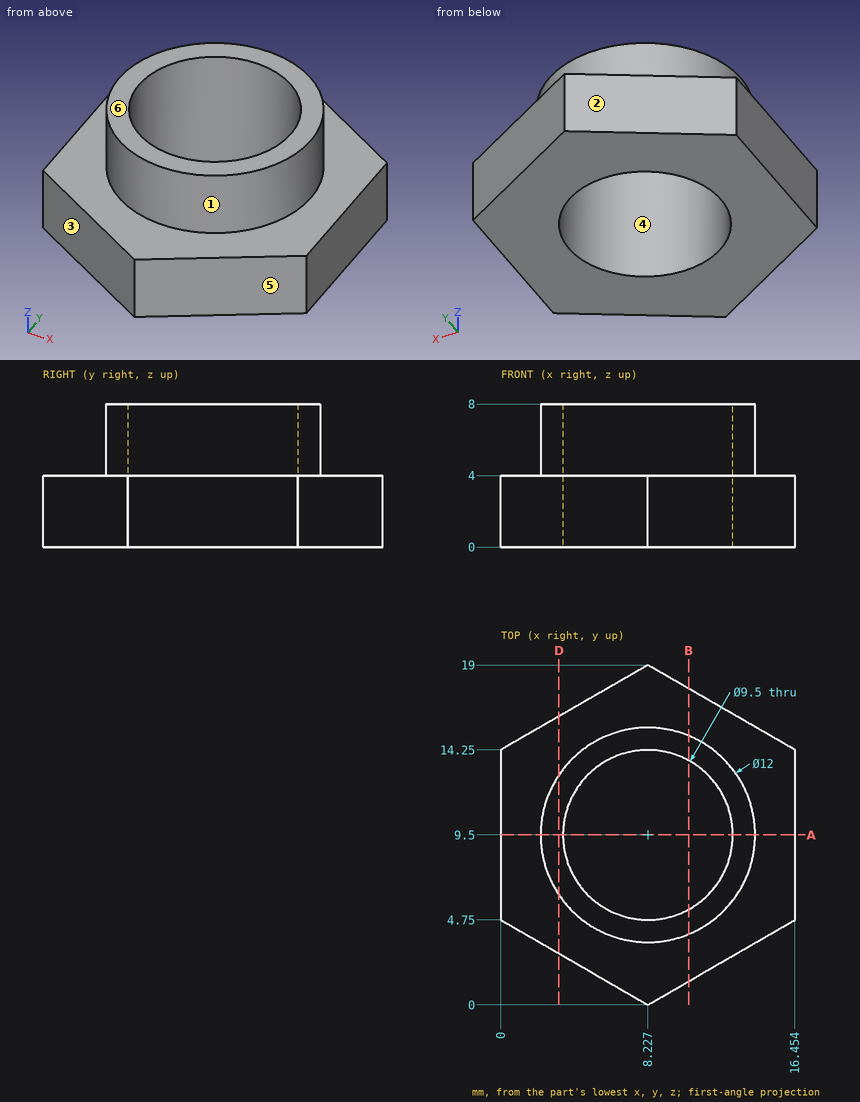
Could you check a few things on this drawing? It's one solid part, dimensions in mm from its lowest x, y, z. A direction names the side the tool comes from. Round coordinates to 2 decimals unless told otherwise and drop trailing zeros. Write each loop counter-clockwise with the first axis right and the second up, starting at its lowest first coordinate (ties: lowest second). Pieces come first, ordered by that corner, then holes.
Q1. Which directions (+Z, -Z, +X, -X, +Y, -Y) give clear straight access to the entire face, cutting with the end or side of a thin tool? Please do the marked faces 1 and 2.
Q2. If we mould it in two halves opening along X, with no side actions, what happens to the marked faces 3, 4, 5 and 6? For each: +X half, -X half, draft (parallel to the pull), parting line (faces both ways), or undercut.
Q3. If we section it at D-D on x = 3.25: Write out the boundary of the cut face in (y, z).
Q4. If we section it at A-A on y = 9.5: Write out the boundary of the cut face in (x, z) (1 decimal).
Q5. If we section it at B-B on x = 10.5: Write out the boundary of the cut face in (y, z).
Q6. Will these pins go through, and if not, where does the flat tip stop? P1, Ø3, axis at x = 9, y = 12, coming from the -Z side; P2, Ø2, axis at x = 13.5, z = 3.5, coming from the +Y side; P3, Ø4, axis at x = 14, y = 12.5, coming from the +Z side; P4, Ø2, axis at x = 12, z = 6.5, coming from the -Y side.
Q7. Please list where these lines run through material, in increasing order: probe 1 along Z at (x, y) = (1.5, 12); probe 2 along Y at (x, z) = (10.5, 2.25); probe 3 along Y at (x, z) = (12.25, 2) (1 decimal).
Answer below:
1. face 1: +Z
1. face 2: +Z, -Z, -X, +Y
2. face 3: -X half
2. face 4: undercut
2. face 5: +X half
2. face 6: draft
3. outline: (2.87, 0) - (16.13, 0) - (16.13, 4) - (12.85, 4) - (12.85, 8) - (6.15, 8) - (6.15, 4) - (2.87, 4) - close
4. outline: (0, 0) - (3.5, 0) - (3.5, 8) - (2.2, 8) - (2.2, 4) - (0, 4) - close; (13, 0) - (16.5, 0) - (16.5, 4) - (14.2, 4) - (14.2, 8) - (13, 8) - close
5. outline: (1.31, 0) - (5.33, 0) - (5.33, 8) - (3.95, 8) - (3.95, 4) - (1.31, 4) - close; (13.67, 0) - (17.69, 0) - (17.69, 4) - (15.05, 4) - (15.05, 8) - (13.67, 8) - close
6. P1: passes through
6. P2: stops at y = 16.53
6. P3: stops at z = 8
6. P4: stops at y = 4.18
7. probe 1: z = 0 to 4
7. probe 2: y = 1.31 to 5.33, 13.67 to 17.69
7. probe 3: y = 2.3 to 7, 12 to 16.7
